```python
from build123d import *

# Parameters (mm, degrees)
SKETCH1_W           = 200
SKETCH1_H           = 200
BOSS_EXTRUDE1_DEPTH = 10
SKETCH2_R           = 5
SKETCH2_R_2         = 2.15
CUT_EXTRUDE1_DEPTH  = 142.774468788
SKETCH3_W           = 20
SKETCH3_H           = 5


with BuildPart() as part:
    # Sketch1 → Boss-Extrude1 (new body)
    with BuildSketch(Plane.XY):
        Rectangle(SKETCH1_W, SKETCH1_H)
    extrude(amount=BOSS_EXTRUDE1_DEPTH)

    # Sketch2 → Cut-Extrude1 (cut, through all)
    with BuildSketch(Plane.XY.offset(10)):
        with Locations((-40, 30)):
            Circle(SKETCH2_R)
        with Locations((40, 30)):
            Circle(SKETCH2_R)
        with Locations((40, -30)):
            Circle(SKETCH2_R)
        with Locations((-40, -30)):
            Circle(SKETCH2_R)
        with Locations((-30, 40)):
            Circle(SKETCH2_R)
        with Locations((30, 40)):
            Circle(SKETCH2_R)
        with Locations((30, -40)):
            Circle(SKETCH2_R)
        with Locations((-30, -40)):
            Circle(SKETCH2_R)
        with Locations((-56.6, 90.4)):
            Circle(SKETCH2_R_2)
        with Locations((-90.4, 56.6)):
            Circle(SKETCH2_R_2)
        with Locations((-90.4, -56.6)):
            Circle(SKETCH2_R_2)
        with Locations((-56.6, -90.4)):
            Circle(SKETCH2_R_2)
        with Locations((56.6, -90.4)):
            Circle(SKETCH2_R_2)
        with Locations((90.4, -56.6)):
            Circle(SKETCH2_R_2)
        with Locations((90.4, 56.6)):
            Circle(SKETCH2_R_2)
        with Locations((56.6, 90.4)):
            Circle(SKETCH2_R_2)
    extrude(amount=-CUT_EXTRUDE1_DEPTH, mode=Mode.SUBTRACT)

    # Sketch3 → Cut-Revolve1 (revolve, cut)
    with BuildSketch(Plane(origin=(0, 0, 0), x_dir=(1, 0, 0), z_dir=(0, 1, 0))):
        with Locations((0, -4.492265688)):
            Rectangle(SKETCH3_W, SKETCH3_H)
    revolve(axis=Axis((0, 0, 354.492265688), (1, 0, 0)), mode=Mode.SUBTRACT)


solid = part.part
```
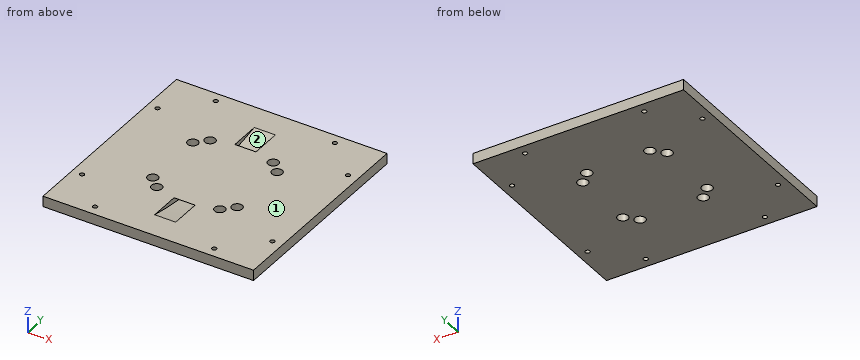
CAD build for the part. Positions are in the model's coordinates, mm. Face numbers are marked on the shaded views. Round coordinates to 2 decimals unless told otherwise and drop trailing zeros. Loops run counter-clockwise (first coordinate to the right, second up) from the corner with the lowest first, then second, coordinate; pieces in that order, holes last. Notation, with made-up numbers: M 46,55.5 L 98,55.5 A15 cw 98,77.5 Z; hole C 31.25,-5 d6. An arc over 180 degrees is marked long. Use a Markdown table: item, result. Add a question column.
(1) Cut at D-D (y = 40). Give the cut face in (x, z).
(2) Cut at B-B (x = 40). Give the cut face in (y, z), and give its area (3 significant figures).
(3) Cut at C-C (y = -8). Give the cut face in (x, z).
(4) Cut at A-A (y = -30). Give the cut face in (x, z).
(5) Drill centre lines: line 1 (Y direction, x = 40, z = 3.75); line 2 (Y direction, x = -56.6, z = 2); line 3 (X direction, y = -88.5, z = 8.5). Where is each one in solid material? Low to high.
(6) Pull direction X, two halves, no side cores. Call the marked faces 1 and 2: +X half, -X half, draft (parallel to the pull), parting line (faces both ways), or undercut.
Geometry says:
| question | item | result |
|---|---|---|
| 1 | outline | M -100,0 L -35,0 L -35,10 L -100,10 Z; M -25,0 L 25,0 L 25,10 L -25,10 Z; M 35,0 L 100,0 L 100,10 L 35,10 Z; hole M -10,4.27 L 10,4.27 L 10,9.3 L -10,9.3 Z |
| 2 | outline | M -100,0 L -35,0 L -35,10 L -100,10 Z; M -25,0 L 25,0 L 25,10 L -25,10 Z; M 35,0 L 100,0 L 100,10 L 35,10 Z |
| 2 | area | 1,800 mm² |
| 3 | outline | M -100,0 L 100,0 L 100,10 L -100,10 Z; hole M -10,2.08 L 10,2.08 L 10,7.08 L -10,7.08 Z |
| 4 | outline | M -100,0 L -45,0 L -45,10 L -100,10 Z; M -35,0 L 35,0 L 35,10 L -35,10 Z; M 45,0 L 100,0 L 100,10 L 45,10 Z; hole M -10,3.27 L 10,3.27 L 10,8.29 L -10,8.29 Z |
| 5 | line 1 | y = -100 to -35, -25 to 25, 35 to 100 |
| 5 | line 2 | y = -100 to -92.55, -88.25 to 88.25, 92.55 to 100 |
| 5 | line 3 | x = -100 to -57.61, -55.59 to 55.59, 57.61 to 100 |
| 6 | face 1 | draft |
| 6 | face 2 | undercut |
